Here's how the part is built. I have some questions about the finished solid (model axes, mm). Round coordinates to 2 decimals unless told otherwise and drop trailing zeros. Write each loop counter-clockwise with the first axis right and the second up, starting at its lowest first coordinate (ties: lowest second). Pieces come first, ordered by that corner, then holes. Notation, with made-up numbers: (5.25, -23) -> (56.25, -23) arc R11 ccw to (56.25, -18) -> close; hole circle Ø4 at (36, -11). An arc over 180 degrees is marked (long way). Answer in a Markdown table with one row per item.
from build123d import *

# Parameters (mm, degrees)
BOSS_EXTRUDE1_DEPTH  = 3.175
SKETCH2_R            = 2.54
CUT_EXTRUDE1_DEPTH   = 3.175
LPATTERN1_COUNT      = 6
LPATTERN1_PITCH      = 25.4
LPATTERN1_COUNT_DIR2 = 2
LPATTERN1_PITCH_DIR2 = 25.4
SKETCH3_R            = 2.54
CUT_EXTRUDE2_DEPTH   = 3.175
LPATTERN2_COUNT      = 2
LPATTERN2_PITCH      = 25.4
LPATTERN2_COUNT_DIR2 = 2
LPATTERN2_PITCH_DIR2 = 25.4


with BuildPart() as part:
    # Sketch1 → Boss-Extrude1 (new body)
    with BuildSketch(Plane(origin=(0, 0, 0), x_dir=(1, 0, 0), z_dir=(0, 1, 0))):
        Polygon((25.4, -25.4), (76.2, -25.4), (76.2, 25.4), (-76.2, 25.4), (-76.2, -25.4), (-25.4, -25.4), (-25.4, -76.2), (25.4, -76.2), align=None)
    extrude(amount=BOSS_EXTRUDE1_DEPTH)

    # Sketch2 → Cut-Extrude1 (cut)
    with BuildSketch(Plane(origin=(0, 3.175, 0), x_dir=(1, 0, 0), z_dir=(0, 1, 0))):
        with Locations(Location((-63.5, 12.7, 0), (0, 0, 270))):
            Circle(SKETCH2_R)
    cut_extrude1 = extrude(amount=-CUT_EXTRUDE1_DEPTH, mode=Mode.SUBTRACT)

    # LPattern1: Cut-Extrude1 6 × 2
    with Locations(*[(i * LPATTERN1_PITCH, 0, j * LPATTERN1_PITCH_DIR2) for i in range(LPATTERN1_COUNT) for j in range(LPATTERN1_COUNT_DIR2) if (i, j) != (0, 0)]):
        add(cut_extrude1, mode=Mode.SUBTRACT)

    # Sketch3 → Cut-Extrude2 (cut)
    with BuildSketch(Plane(origin=(0, 3.175, 0), x_dir=(1, 0, 0), z_dir=(0, 1, 0))):
        with Locations(Location((-12.7, -63.5, 0), (0, 0, 270))):
            Circle(SKETCH3_R)
    cut_extrude2 = extrude(amount=-CUT_EXTRUDE2_DEPTH, mode=Mode.SUBTRACT)

    # LPattern2: Cut-Extrude2 2 × 2
    with Locations(*[(i * LPATTERN2_PITCH, 0, -j * LPATTERN2_PITCH_DIR2) for i in range(LPATTERN2_COUNT) for j in range(LPATTERN2_COUNT_DIR2) if (i, j) != (0, 0)]):
        add(cut_extrude2, mode=Mode.SUBTRACT)


solid = part.part
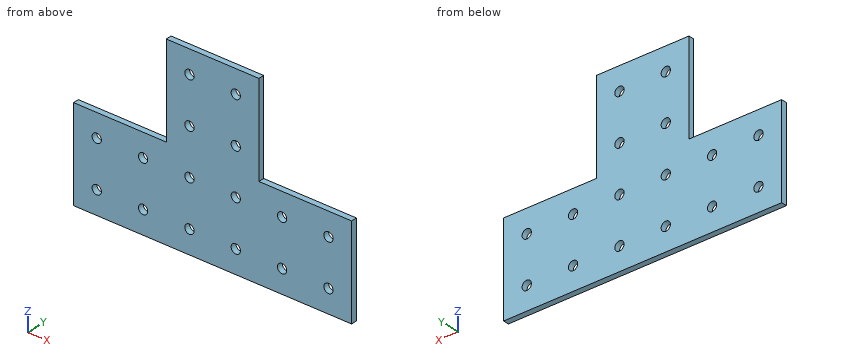
1) I want a section at A-A, the plane y = 1.4. Count the separate pieces of the cut face and the enclosed holes in it, and give its area (4 significant figures).
Response:
| item | result |
|---|---|
| separate pieces | 1 |
| enclosed holes | 16 |
| area | 10,000 mm^2 |
2) For pin 1 (1.6 mm diameter, centred on y = 1, z = 56, fed in from +X), with a flat end and sliding along its axis, tell me the tip position at first contact or that it passes through.
Response:
| item | result |
|---|---|
| pin 1 | stops at x = 25.4 |
3) I want a section at C-C, the plane x = -12.7. List the corners of the cut face in (y, z) for me (3 decimals), and give its area (3 significant figures).
Response:
| item | result |
|---|---|
| outline | (0, -25.4) -> (3.175, -25.4) -> (3.175, -15.24) -> (0, -15.24) -> close; (0, -10.16) -> (3.175, -10.16) -> (3.175, 10.16) -> (0, 10.16) -> close; (0, 15.24) -> (3.175, 15.24) -> (3.175, 35.56) -> (0, 35.56) -> close; (0, 40.64) -> (3.175, 40.64) -> (3.175, 60.96) -> (0, 60.96) -> close; (0, 66.04) -> (3.175, 66.04) -> (3.175, 76.2) -> (0, 76.2) -> close |
| area | 258 mm^2 |
4) I need wall thicknesses on line 1 (Z direction, x = 38.1, y = 2); line 2 (X direction, y = 2.9, z = 64.5); line 3 (Z direction, x = 65.5, y = 2.7). Which ranges of each line are inside material? Lowest first, please. Write a range as [from, to].
Response:
| item | result |
|---|---|
| line 1 | z = [-25.4, -15.24], [-10.16, 10.16], [15.24, 25.4] |
| line 2 | x = [-25.4, -15.03], [-10.37, 10.37], [15.03, 25.4] |
| line 3 | z = [-25.4, -14.27], [-11.13, 11.13], [14.27, 25.4] |
5) I want a section at B-B, the plane z = 38.1. List the corners of the cut face in (x, y) for me (3 decimals).
Response:
| item | result |
|---|---|
| outline | (-25.4, 0) -> (-15.24, 0) -> (-15.24, 3.175) -> (-25.4, 3.175) -> close; (-10.16, 0) -> (10.16, 0) -> (10.16, 3.175) -> (-10.16, 3.175) -> close; (15.24, 0) -> (25.4, 0) -> (25.4, 3.175) -> (15.24, 3.175) -> close |
6) I want a section at D-D, the plane x = 63.5. List the corners of the cut face in (y, z) for me (3 decimals), and give its area (3 significant figures).
Response:
| item | result |
|---|---|
| outline | (0, -25.4) -> (3.175, -25.4) -> (3.175, -15.24) -> (0, -15.24) -> close; (0, -10.16) -> (3.175, -10.16) -> (3.175, 10.16) -> (0, 10.16) -> close; (0, 15.24) -> (3.175, 15.24) -> (3.175, 25.4) -> (0, 25.4) -> close |
| area | 129 mm^2 |
